from build123d import *

# Parameters (mm, degrees)
F1_DEPTH = 1
F3_DEPTH = 10
F4_D     = 3
F4_DEPTH = 5
F6_DEPTH = 25


with BuildPart() as f1:
    # F0 (on Top) → F1 (new body)
    with BuildSketch(Plane.XY):
        with BuildLine():
            Line((12, 13.5), (-12, 13.5))
            ThreePointArc((-12, 13.5), (-13.06066, 13.06066), (-13.5, 12))
            Line((-13.5, 12), (-13.5, -12))
            ThreePointArc((-13.5, -12), (-13.06066, -13.06066), (-12, -13.5))
            Line((-12, -13.5), (12, -13.5))
            ThreePointArc((12, -13.5), (13.06066, -13.06066), (13.5, -12))
            Line((13.5, -12), (13.5, 12))
            ThreePointArc((13.5, 12), (13.06066, 13.06066), (12, 13.5))
        make_face()
    extrude(amount=F1_DEPTH)

    # F2 (on Right) → F3 (join, symmetric)
    with BuildSketch(Plane.YZ):
        Polygon((6.433479, 4.475368), (3.479055, 3.954423), (1.884076, 13), (-1.115924, 13), (-1.115924, 1), (4, 1), (7.04628, 1), align=None)
    extrude(amount=F3_DEPTH, both=True)

    # F4
    with Locations(Plane(origin=(0, 0, 0), x_dir=(1, 0, 0), z_dir=(0, 0, -1))):
        with Locations((10, -10), (-10, -10), (-10, 10), (10, 10)):
            Hole(F4_D / 2, depth=F4_DEPTH)

    # F5 (on face) → F6 (cut)
    with BuildSketch(Plane.XY.offset(1)):
        with BuildLine():
            Line((-1.615174, -2.115924), (-10, -2.115924))
            Line((-10, -2.115924), (-10, -7.5))
            ThreePointArc((-10, -7.5), (-9.391612, -7.575157), (-8.819804, -7.796109))
            Line((-8.819804, -7.796109), (-1.615174, -2.115924))
        make_face()
        with BuildLine():
            ThreePointArc((-7.581547, -9.366688), (-7.52047, -9.68073), (-7.5, -10))
            Line((-7.5, -10), (7.5, -10))
            ThreePointArc((7.5, -10), (7.52047, -9.68073), (7.581547, -9.366688))
            Line((7.581547, -9.366688), (0, -3.389339))
            Line((0, -3.389339), (-7.581547, -9.366688))
        make_face()
        with BuildLine():
            ThreePointArc((8.819804, -7.796109), (9.391612, -7.575157), (10, -7.5))
            Line((10, -7.5), (10, -2.115924))
            Line((10, -2.115924), (1.615174, -2.115924))
            Line((1.615174, -2.115924), (8.819804, -7.796109))
        make_face()
    extrude(amount=-F6_DEPTH, mode=Mode.SUBTRACT)


solid = f1.part
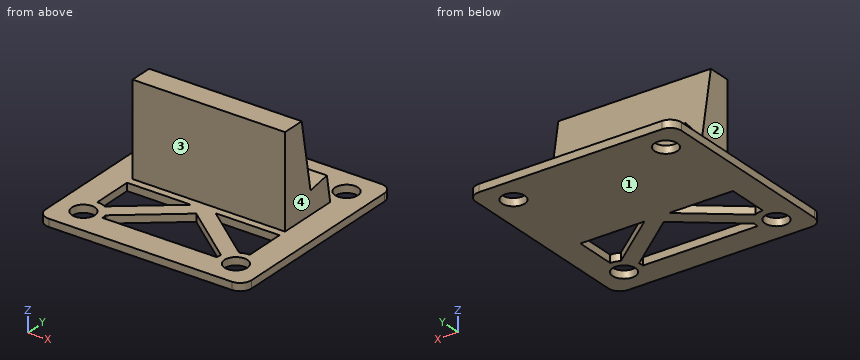
Design review of the part built by this model. Coordinates are the model's own, in mm. Face numbers are marked on the shaded views. A direction names the side the tool comes from. Coordinates: 2 decimals unless noted, no trailing zeros. Loops run counter-clockwise (first coordinate to the right, second up) from the corner with the lowest first, then second, coordinate; pieces in that order, holes last. Notation, with made-up numbers: (7, -23.5) - (35, -23.5) arc R24 cw to (35, -5.5) - close; hole circle Ø11 at (10.25, 23). An arc over 180 degrees is marked (long way). Use CSV: the item, a comma, the result in double quotes. Start each with the question number.
1. Clearance check with flat-ended pins moving along their axes: pin 1 (1.5 mm diameter, centred on x = -5, y = -5, fed in from -Z); pin 2 (2 mm diameter, centred on y = -2.5, z = 7.5, fed in from -X); pin 3 (4 mm diameter, centred on y = 4, z = 9, fed in from -X); pin 4 (3.5 mm diameter, centred on x = 0.5, z = 7.5, fed in from -Y). State where each tip first meets the part, or that it passes through.
2. Add section A-A on y = 10. Give the boundary of the cut face in (x, z).
3. For the marked faces 1, 2, 3 and 4, list the 3-axis set-ups (+Z, -Z, +X, -X, +Y, -Y) from which the entire face can be reached by the end or side of a thin tool; tool diameter is ignored.
4. Add section C-C on y = -2.5. Give the boundary of the cut face in (x, z).
5. Add section D-D on z = 11.5. Give the boundary of the cut face in (x, y).
6. Add section B-B on y = 5.75. Give the boundary of the cut face in (x, z), plus the area to 3 significant figures.
7. To check wall thickness, follow probe 1 along X at (y, z) = (10, 0.3); probe 2 along Z at (x, y) = (-4.5, -5.75); probe 3 along Z at (x, y) = (-6.25, 5.5). State the ranges of each line that lie inside material, in increasing order.
Resolved:
1,pin 1,"z = 0"
1,pin 2,"through"
1,pin 3,"x = -10"
1,pin 4,"y = -1.12"
2,outline,"(-13.5, 0) - (-11.5, 0) - (-11.5, 1) - (-13.5, 1) - close; (-8.5, 0) - (8.5, 0) - (8.5, 1) - (-8.5, 1) - close; (11.5, 0) - (13.5, 0) - (13.5, 1) - (11.5, 1) - close"
3,face 1,"-Z, +X, -X, +Y, -Y"
3,face 2,"+Z, -X, +Y, -Y"
3,face 3,"+Z, +X, -X, -Y"
3,face 4,"+Z, +X, +Y, -Y"
4,outline,"(-13.5, 0) - (-10, 0) - (-10, 1) - (-13.5, 1) - close; (-2.1, 0) - (2.1, 0) - (2.1, 1) - (-2.1, 1) - close; (10, 0) - (13.5, 0) - (13.5, 1) - (10, 1) - close"
5,outline,"(-10, -1.12) - (10, -1.12) - (10, 2.15) - (-10, 2.15) - close"
6,outline,"(-13.5, 0) - (13.5, 0) - (13.5, 1) - (10, 1) - (10, 4.35) - (-10, 4.35) - (-10, 1) - (-13.5, 1) - close"
6,area,"94.1 mm2"
7,probe 1,"-13.5 to -11.5, -8.5 to 8.5, 11.5 to 13.5"
7,probe 2,"0 to 1"
7,probe 3,"0 to 4.31"
